from build123d import *

# Parameters (mm, degrees)
BOSS_EXTRUDE1_DEPTH     = 23
SKETCH2_R               = 1.55
CUT_EXTRUDE1_DEPTH      = 30
BOSS_EXTRUDE2_DEPTH     = 10
SKETCH5_R               = 4
CUT_EXTRUDE3_DEPTH      = 70
ESQUISSE1_R             = 4.15
ENL_V_MAT_EXTRU_1_DEPTH = 3


with BuildPart() as part:
    # Sketch1 → Boss-Extrude1 (new body)
    with BuildSketch(Plane.XY):
        with BuildLine():
            Line((-10, -4.786331479), (-10, 25.213668521))
            ThreePointArc((-10, 25.213668521), (0, 35.213668521), (10, 25.213668521))
            Line((10, 25.213668521), (10, -4.786331479))
            ThreePointArc((10, -4.786331479), (0, -14.786331479), (-10, -4.786331479))
        make_face()
    extrude(amount=BOSS_EXTRUDE1_DEPTH)

    # Sketch2 → Cut-Extrude1 (cut)
    with BuildSketch(Plane.XY.offset(23)):
        with Locations((0, 25.213668521)):
            Circle(SKETCH2_R)
        with Locations((0, -4.786331479)):
            Circle(SKETCH2_R)
    extrude(amount=-CUT_EXTRUDE1_DEPTH, mode=Mode.SUBTRACT)

    # Sketch3 → Boss-Extrude2 (add)
    with BuildSketch(Plane(origin=(0, 0, 0), x_dir=(-1, 0, 0), z_dir=(0, 0, -1))):
        with BuildLine():
            Line((-15, 25.213668521), (-15, -4.786331479))
            ThreePointArc((-15, -4.786331479), (0, -19.786331479), (15, -4.786331479))
            Line((15, -4.786331479), (15, 25.213668521))
            ThreePointArc((15, 25.213668521), (0, 40.213668521), (-15, 25.213668521))
        make_face()
        with BuildLine():
            Line((-10, 25.213668521), (-10, -4.786331479))
            ThreePointArc((-10, -4.786331479), (0, -14.786331479), (10, -4.786331479))
            Line((10, -4.786331479), (10, 25.213668521))
            ThreePointArc((10, 25.213668521), (0, 35.213668521), (-10, 25.213668521))
        make_face(mode=Mode.SUBTRACT)
    extrude(amount=-BOSS_EXTRUDE2_DEPTH)

    # Sketch5 → Cut-Extrude3 (cut)
    with BuildSketch(Plane.XY.offset(23)):
        with Locations((0, 10.213668521)):
            Circle(SKETCH5_R)
    extrude(amount=-CUT_EXTRUDE3_DEPTH, mode=Mode.SUBTRACT)

    # Esquisse1 → Enlèv. mat.-Extru.1 (cut)
    with BuildSketch(Plane(origin=(0, 0, 0), x_dir=(-1, 0, 0), z_dir=(0, 0, -1))):
        with Locations((0, 25.213668521)):
            Circle(ESQUISSE1_R)
        with Locations((0, -4.786331479)):
            Circle(ESQUISSE1_R)
    extrude(amount=-ENL_V_MAT_EXTRU_1_DEPTH, mode=Mode.SUBTRACT)


solid = part.part
Verification items for the finished model (mm, model axes). A direction names the side the tool comes from. Round coordinates to 2 decimals unless told otherwise and drop trailing zeros. Order: outer loops, then holes, each group sorted by start corner. A loop starts at its lowest first (then second) coordinate and runs counter-clockwise, first axis right, second up. Notation, with made-up numbers: (68, 86.25) -> (75, 86.25) arc R14 cw to (75, 108.25) -> close; hole circle Ø10 at (2.5, 75.5). An arc over 180 degrees is marked (long way). Put each result on its own line as item: value.
1) Mould release check, pull along Y, two halves, no side actions. Record for faces 1 (the cylindrical face through (-0.33, 40.21, 4.93)), 2 (the flat face through (15, 10, 5)), 3 (the flat face through (-2, 25, 3)): +Y half, -Y half, draft (parallel to the pull), parting line (faces both ways), or undercut.
Final values:
face 1: +Y half
face 2: draft
face 3: undercut
2) Section check A-A (x = 0). Record the cut outline in (y, z).
Final values:
outline: (-19.79, 0) -> (-8.94, 0) -> (-8.94, 3) -> (-6.34, 3) -> (-6.34, 23) -> (-14.79, 23) -> (-14.79, 10) -> (-19.79, 10) -> close; (-3.24, 3) -> (-0.64, 3) -> (-0.64, 0) -> (6.21, 0) -> (6.21, 23) -> (-3.24, 23) -> close; (14.21, 0) -> (21.06, 0) -> (21.06, 3) -> (23.66, 3) -> (23.66, 23) -> (14.21, 23) -> close; (26.76, 3) -> (29.36, 3) -> (29.36, 0) -> (40.21, 0) -> (40.21, 10) -> (35.21, 10) -> (35.21, 23) -> (26.76, 23) -> close
3) Set-up check for faces 4 (the cylindrical face through (0.54, 29.33, 1.48)), 5 (the flat face through (-10, 10, 16)), 6 (the flat face through (10.2, 10.6, 10)), 7 (the cylindrical face through (0.22, -14.784, 16.409)), 8 (the cylindrical face through (-0.22, 35.21, 16.41)): record each of +Z, -Z, +X, -X, +Y, -Y from which the full face is reachable in a straight line by a thin tool's end or side.
Final values:
face 4: -Z
face 5: +Z, -X, +Y, -Y
face 6: +Z
face 7: +Z, -Y
face 8: +Z, +Y
4) Section check C-C (z = 2). Record the cut outline in (x, y).
Final values:
outline: (-15, -4.79) arc R15 ccw to (15, -4.79) -> (15, 25.21) arc R15 ccw to (-15, 25.21) -> close; hole circle Ø8.3 at (0, -4.79); hole circle Ø8.3 at (0, 25.21); hole circle Ø8 at (0, 10.21)
5) Section check D-D (y = 18.5). Record the cut outline in (x, z).
Final values:
outline: (-15, 0) -> (15, 0) -> (15, 10) -> (10, 10) -> (10, 23) -> (-10, 23) -> (-10, 10) -> (-15, 10) -> close
6) Material ranges on line 1 (Y direction, x = 0, z = 12.5); line 2 (Y direction, x = 0, z = 1.1); line 3 (X direction, y = 10, z = 20), recorded low to high.
Final values:
line 1: y = -14.79 to -6.34, -3.24 to 6.21, 14.21 to 23.66, 26.76 to 35.21
line 2: y = -19.79 to -8.94, -0.64 to 6.21, 14.21 to 21.06, 29.36 to 40.21
line 3: x = -10 to -3.99, 3.99 to 10
7) Depth check by flat-ended pin: pin 1 (9.5 mm diameter, centred on x = 0, y = 25.21, fed in from +Z); pin 2 (1 mm diameter, centred on y = 4.5, z = 13, fed in from -X); pin 3 (4 mm diameter, centred on x = 0, y = -4.79, fed in from -Z); pin 4 (5 mm diameter, centred on x = 4, z = 5.5, fed in from +Y). Enter the tip coordinate at first touch or a pass-through.
Final values:
pin 1: stops at z = 23
pin 2: stops at x = -10
pin 3: stops at z = 3
pin 4: stops at y = 40.14
8) Section check B-B (y = -5.5). Record the cut outline in (x, z).
Final values:
outline: (-14.98, 0) -> (-4.09, 0) -> (-4.09, 3) -> (-1.38, 3) -> (-1.38, 23) -> (-9.97, 23) -> (-9.97, 10) -> (-14.98, 10) -> close; (1.38, 3) -> (4.09, 3) -> (4.09, 0) -> (14.98, 0) -> (14.98, 10) -> (9.97, 10) -> (9.97, 23) -> (1.38, 23) -> close
